Geometry check sheet. Reference: the model listing, model coordinates, mm. Face numbers are marked on the shaded views. A direction names the side the tool comes from. Round coordinates to 2 decimals unless told otherwise and drop trailing zeros. Loops run counter-clockwise (first coordinate to the right, second up) from the corner with the lowest first, then second, coordinate; pieces in that order, holes last. Notation, with made-up numbers: (7.25, 65) - (57.25, 65) arc R34 ccw to (57.25, 102) - close; hole circle Ø11 at (54, 74.25). An arc over 180 degrees is marked (long way). Answer as CSV lines item,"result". Start each with the question number.
1) Draft check along X on the marked faces 1, 2 and 3. Enter one of: released by +X, released by -X, zero draft, split by the parting line, or undercut.
2) Cross-section at A-A on y = 300. Record the boundary of the cut face in (x, z), and give its area (3 significant figures).
3) Cross-section at B-B on z = 46.5. Record the boundary of the cut face in (x, y).
4) Access from +Z, -Z, +X, -X, +Y, -Y to the whole of each face (thin tool, end or side, straight path). Record for the marked faces 4 and 5.
5) Thickness scan on line 1 along X through (y, z) = (343, 8); line 2 along Y through (x, z) = (535.5, 62); line 3 along X through (y, z) = (269.5, 10). Record the ranges inside material, lowest first.
6) Cross-section at C-C on x = 579. Record the boundary of the cut face in (y, z).
Autodesk Fusion 360 part; units mm, degrees
sketch "スケッチ1" plane through (0, 0, 0) normal (0, 0, 1) x (1, 0, 0)
  arc A0 (506.3587, 411.6011) -> (492.8587, 398.1011) centre (506.3587, 398.1011) ccw
  arc A1 (506.3587, 407.1011) -> (497.3587, 398.1011) centre (506.3587, 398.1011) ccw
  arc A2 (642.8587, 398.1011) -> (629.3587, 411.6011) centre (629.3587, 398.1011) ccw
  arc A3 (638.3587, 398.1011) -> (629.3587, 407.1011) centre (629.3587, 398.1011) ccw
  line L0 (506.3587, 261.6011) -> (629.3587, 261.6011)
  line L1 (506.3587, 266.1011) -> (629.3587, 266.1011)
  arc A4 (492.8587, 275.1011) -> (506.3587, 261.6011) centre (506.3587, 275.1011) ccw
  arc A5 (497.3587, 275.1011) -> (506.3587, 266.1011) centre (506.3587, 275.1011) ccw
  line L2 (492.8587, 398.1011) -> (492.8587, 275.1011)
  line L3 (497.3587, 398.1011) -> (497.3587, 275.1011)
  arc A6 (629.3587, 261.6011) -> (642.8587, 275.1011) centre (629.3587, 275.1011) ccw
  arc A7 (629.3587, 266.1011) -> (638.3587, 275.1011) centre (629.3587, 275.1011) ccw
  line L4 (638.3587, 275.1011) -> (638.3587, 398.1011)
  line L5 (642.8587, 275.1011) -> (642.8587, 398.1011)
  line L6 (629.3587, 411.6011) -> (506.3587, 411.6011)
  line L7 (629.3587, 407.1011) -> (506.3587, 407.1011)
  point P0 (567.8587, 336.6011)
extrude "押し出し1" add sketch "スケッチ1" along normal blind 100
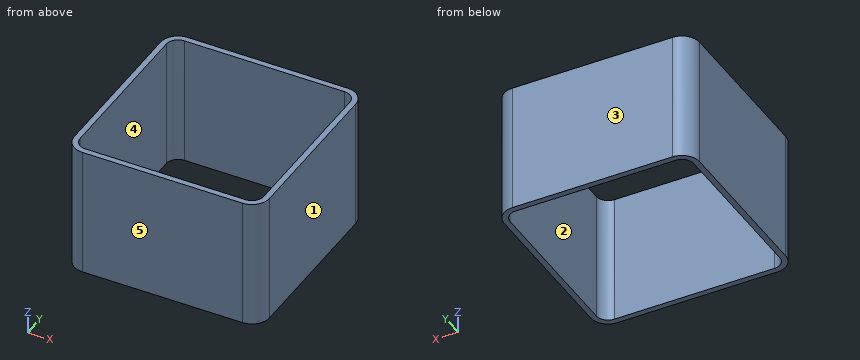
Answer block:
1,face 1,"released by +X"
1,face 2,"undercut"
1,face 3,"zero draft"
2,outline,"(492.86, 0) - (497.36, 0) - (497.36, 100) - (492.86, 100) - close; (638.36, 0) - (642.86, 0) - (642.86, 100) - (638.36, 100) - close"
2,area,"900 mm^2"
3,outline,"(492.86, 275.1) arc R13.5 ccw to (506.36, 261.6) - (629.36, 261.6) arc R13.5 ccw to (642.86, 275.1) - (642.86, 398.1) arc R13.5 ccw to (629.36, 411.6) - (506.36, 411.6) arc R13.5 ccw to (492.86, 398.1) - close; hole (497.36, 275.1) arc R9 ccw to (506.36, 266.1) - (629.36, 266.1) arc R9 ccw to (638.36, 275.1) - (638.36, 398.1) arc R9 ccw to (629.36, 407.1) - (506.36, 407.1) arc R9 ccw to (497.36, 398.1) - close"
4,face 4,"+Z, -Z"
4,face 5,"+Z, -Z, +X, -X, -Y"
5,line 1,"x = 492.86 to 497.36, 638.36 to 642.86"
5,line 2,"y = 261.6 to 266.1, 407.1 to 411.6"
5,line 3,"x = 494.08 to 499.31, 636.4 to 641.64"
6,outline,"(261.6, 0) - (266.1, 0) - (266.1, 100) - (261.6, 100) - close; (407.1, 0) - (411.6, 0) - (411.6, 100) - (407.1, 100) - close"
